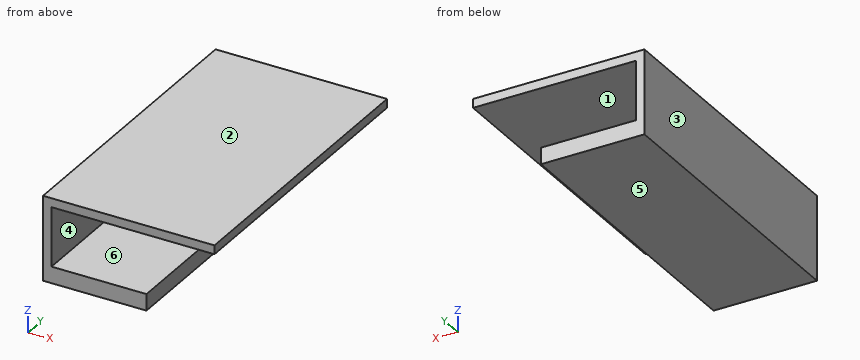
```python
from build123d import *

# Parameters (mm, degrees)
SKETCH2_W           = 106
SKETCH2_H           = 106
SKETCH2_R           = 4
SKETCH2_R_2         = 6
BOSS_EXTRUDE1_DEPTH = 25
SKETCH3_W           = 106
SKETCH3_H           = 106
SKETCH3_W_2         = 100
SKETCH3_H_2         = 100
BOSS_EXTRUDE2_DEPTH = 20
SKETCH5_W           = 3
SKETCH5_H           = 23
BOSS_EXTRUDE3_DEPTH = 20
SKETCH7_W           = 20
SKETCH7_H           = 3
BOSS_EXTRUDE4_DEPTH = 20
SKETCH9_R           = 9.905763918
CUT_EXTRUDE1_DEPTH  = 10
SKETCH10_W          = 10
SKETCH10_H          = 4
BOSS_EXTRUDE5_DEPTH = 10
SKETCH11_W          = 10
SKETCH11_H          = 4
BOSS_EXTRUDE6_DEPTH = 10
FILLET2_RADIUS      = 5
FILLET2_LENGTH      = 4
FILLET3_R           = 5
FILLET4_R           = 5
FILLET5_R           = 5
SKETCH13_R          = 1.6
CUT_EXTRUDE2_DEPTH  = 163.397660082
SKETCH14_W          = 35.96051594
SKETCH14_H          = 7.693498276
CUT_EXTRUDE3_DEPTH  = 30
BOSS_EXTRUDE7_DEPTH = 100
SKETCH21_W          = 151.44967638
SKETCH21_H          = 134.741704964
CUT_EXTRUDE6_DEPTH  = 187.257885739


with BuildPart() as part:
    # Sketch2 → Boss-Extrude1 (new body)
    with BuildSketch(Plane(origin=(0, 0, 0), x_dir=(1, 0, 0), z_dir=(0, 1, 0))):
        with Locations((53, 53)):
            Rectangle(SKETCH2_W, SKETCH2_H)
        with Locations(Location((18, 15, 0), (0, 0, 270))):
            Circle(SKETCH2_R, mode=Mode.SUBTRACT)
        with Locations(Location((92, 13.5, 0), (0, 0, 270))):
            Circle(SKETCH2_R_2, mode=Mode.SUBTRACT)
    extrude(amount=BOSS_EXTRUDE1_DEPTH)

    # Sketch3 → Boss-Extrude2 (add)
    with BuildSketch(Plane(origin=(0, 25, 0), x_dir=(1, 0, 0), z_dir=(0, 1, 0))):
        with Locations((53, 53)):
            Rectangle(SKETCH3_W, SKETCH3_H)
        with Locations((53, 53)):
            Rectangle(SKETCH3_W_2, SKETCH3_H_2, mode=Mode.SUBTRACT)
    extrude(amount=BOSS_EXTRUDE2_DEPTH)

    # Sketch5 → Boss-Extrude3 (add)
    with BuildSketch(Plane(origin=(0, 25, 0), x_dir=(1, 0, 0), z_dir=(0, 1, 0))):
        Polygon((3, 28), (3, 25), (32, 25), (32, 23), (35, 23), (35, 43), (32, 43), (32, 28), align=None)
        Polygon((83, 52.5), (83, 26.5), (76, 26.5), (76, 3), (73, 3), (73, 29.5), (80, 29.5), (80, 49.5), (73, 49.5), (73, 52.5), align=None)
        Polygon((3, 63), (3, 60), (25, 60), (25, 80), (22, 80), (22, 63), align=None)
        with Locations((59.5, 14.5)):
            Rectangle(SKETCH5_W, SKETCH5_H)
    extrude(amount=BOSS_EXTRUDE3_DEPTH)

    # Sketch7 → Boss-Extrude4 (add)
    with BuildSketch(Plane(origin=(0, 25, 0), x_dir=(1, 0, 0), z_dir=(0, 1, 0))):
        Polygon((50, 70.496538655), (53, 70.496538655), (53, 73.496538655), (53, 83.496538655), (50, 83.496538655), align=None)
        with Locations((63, 71.996538655)):
            Rectangle(SKETCH7_W, SKETCH7_H)
        Polygon((73, 70.496538655), (73, 52.5), (76, 52.5), (76, 82.5), (73, 82.5), (73, 73.496538655), align=None)
    extrude(amount=BOSS_EXTRUDE4_DEPTH)

    # Sketch9 → Cut-Extrude1 (cut)
    with BuildSketch(Plane(origin=(0, 25, 0), x_dir=(1, 0, 0), z_dir=(0, 1, 0))):
        with Locations(Location((92, 13.5, 0), (0, 0, 270))):
            Circle(SKETCH9_R)
    extrude(amount=-CUT_EXTRUDE1_DEPTH, mode=Mode.SUBTRACT)

    # Sketch10 → Boss-Extrude5 (add)
    with BuildSketch(Plane.XY):
        with Locations((53, 2)):
            Rectangle(SKETCH10_W, SKETCH10_H)
    extrude(amount=BOSS_EXTRUDE5_DEPTH)

    # Sketch11 → Boss-Extrude6 (add)
    with BuildSketch(Plane(origin=(0, 0, -106), x_dir=(-1, 0, 0), z_dir=(0, 0, -1))):
        with Locations((-53, 2)):
            Rectangle(SKETCH11_W, SKETCH11_H)
    extrude(amount=BOSS_EXTRUDE6_DEPTH)

    # Fillet2: full round fillet: the end face becomes a half cylinder, R = half its width
    fillet2_face = Plane((53, 2, -116), x_dir=(0, -1, 0), z_dir=(0, 0, -1))  # on the end face: x along it, z out of the body
    fillet2_slab = fillet2_face.offset(-FILLET2_RADIUS / 2) * Box(FILLET2_LENGTH, 2 * FILLET2_RADIUS, FILLET2_RADIUS, mode=Mode.PRIVATE)  # the body's end, R deep
    fillet2_round = Plane((53, 2, -111), x_dir=(0, 0, -1), z_dir=(0, -1, 0)) * Cylinder(FILLET2_RADIUS, FILLET2_LENGTH, mode=Mode.PRIVATE)  # its axis R under the face
    add(fillet2_slab - fillet2_round, mode=Mode.SUBTRACT)

    # Fillet3
    fillet3_edges = [part.edges().sort_by_distance(p)[0] for p in [
        (48, 2, -106),
        (58, 2, -106),
    ]]
    fillet(fillet3_edges, radius=FILLET3_R - 0.0001)  # a hair under: the kernel refuses the full size

    # Fillet4
    fillet4_edges = [part.edges().sort_by_distance(p)[0] for p in [
        (48, 2, 0),
        (58, 2, 0),
    ]]
    fillet(fillet4_edges, radius=FILLET4_R)

    # Fillet5
    fillet5_edges = [part.edges().sort_by_distance(p)[0] for p in [
        (48, 2, 10),
        (58, 2, 10),
    ]]
    fillet(fillet5_edges, radius=FILLET5_R - 0.0001)  # a hair under: the kernel refuses the full size

    # Sketch13 → Cut-Extrude2 (cut, through all)
    with BuildSketch(Plane(origin=(0, 4, 0), x_dir=(1, 0, 0), z_dir=(0, 1, 0))):
        with Locations(Location((53, -5, 0), (0, 0, 180))):
            Circle(SKETCH13_R)
        with Locations(Location((53, 111, 0), (0, 0, 180))):
            Circle(SKETCH13_R)
    extrude(amount=-CUT_EXTRUDE2_DEPTH, mode=Mode.SUBTRACT)

    # Sketch14 → Cut-Extrude3 (cut)
    with BuildSketch(Plane.XY):
        with Locations((88.01974203, 3.846749138)):
            Rectangle(SKETCH14_W, SKETCH14_H)
    extrude(amount=-CUT_EXTRUDE3_DEPTH, mode=Mode.SUBTRACT)

    # Sketch15 → Boss-Extrude7 (add)
    with BuildSketch(Plane(origin=(0, 45, 0), x_dir=(1, 0, 0), z_dir=(0, 1, 0))):
        Polygon((0, 28.5668375), (0, 0), (2.876085753, 0), (58, 0), (58, 3), (2.876085753, 3), (2.876085753, 23), (35, 23), (35, 28.5668375), align=None)
    extrude(amount=BOSS_EXTRUDE7_DEPTH)

    # Sketch21 → Cut-Extrude6 (cut, through all)
    with BuildSketch(Plane(origin=(0, 45, 0), x_dir=(1, 0, 0), z_dir=(0, 1, 0))):
        with Locations((51.832238557, 52.101721967)):
            Rectangle(SKETCH21_W, SKETCH21_H)
    extrude(amount=-CUT_EXTRUDE6_DEPTH, mode=Mode.SUBTRACT)


solid = part.part
```
Input: part model. Units: mm. Frame: model coordinates. Face numbers are marked on the shaded views. A direction names the side the tool comes from. Round coordinates to 2 decimals unless told otherwise and drop trailing zeros. Order: outer loops, then holes, each group sorted by start corner. A loop starts at its lowest first (then second) coordinate and runs counter-clockwise, first axis right, second up. Notation, with made-up numbers: (87.25, 0) - (95.25, 0) arc R10 ccw to (95.25, 15) - close; hole circle Ø9 at (16.5, 77). An arc over 180 degrees is marked (long way). Answer in a Markdown table with one row per item.
Item 1: Line query: line 1 (Z direction, x = 3.5, y = 77); line 2 (X direction, y = 60.5, z = -11.75); line 3 (Z direction, x = 52.5, y = 109.5). Output: solid intervals per line, ascending.
Model answer:
| item | result |
|---|---|
| line 1 | z = -28.57 to -23, -3 to 0 |
| line 2 | x = 0 to 2.88 |
| line 3 | z = -3 to 0 |
Item 2: Section query B-B (y = 90.5). Return the cut outline in (x, z), then the cut area to 3 significant figures.
Model answer:
| item | result |
|---|---|
| outline | (0, -28.57) - (35, -28.57) - (35, -23) - (2.88, -23) - (2.88, -3) - (58, -3) - (58, 0) - (0, 0) - close |
| area | 426 mm² |
Item 3: Mould query, pull axis Z, two halves, no side actions, for the marked faces 1, 2, 3 and 4. Classes: released by +Z, released by -Z, zero draft, split by the parting line, or undercut.
Model answer:
| item | result |
|---|---|
| face 1 | undercut |
| face 2 | released by +Z |
| face 3 | zero draft |
| face 4 | undercut |
Item 4: Reachability of the marked faces 5 and 6 from +Z, -Z, +X, -X, +Y, -Y: full face, straight path, thin tool, end or side. Return the list, or none.
Model answer:
| item | result |
|---|---|
| face 5 | -Z, +X, -X, +Y, -Y |
| face 6 | +X, +Y, -Y |
Item 5: Section query D-D (x = 41.5). Return the cut outline in (y, z).
Model answer:
| item | result |
|---|---|
| outline | (45, -3) - (145, -3) - (145, 0) - (45, 0) - close |
Item 6: Pin query (flat end, axial travel): pin 1 (3 mm diameter, centred on y = 109.5, z = -13, fed in from +X); pin 2 (6 mm diameter, centred on y = 87, z = -24.5, fed in from +X); pin 3 (1 mm diameter, centred on x = 49.5, y = 94, fed in from -Z); pin 4 (1.5 mm diameter, centred on x = 25.5, z = -5, fed in from +Y). Return the tip coordinate at first contact, or that it passes through.
Model answer:
| item | result |
|---|---|
| pin 1 | stops at x = 2.88 |
| pin 2 | stops at x = 35 |
| pin 3 | stops at z = -3 |
| pin 4 | passes through |
Item 7: Section query C-C (z = -11.5). Return the cut outline in (x, y), then the cut area to 3 significant figures.
Model answer:
| item | result |
|---|---|
| outline | (0, 45) - (2.88, 45) - (2.88, 145) - (0, 145) - close |
| area | 288 mm² |
Item 8: Section query A-A (x = 27). Return the cut outline in (y, z), then the cut area to 3 significant figures.
Model answer:
| item | result |
|---|---|
| outline | (45, -28.57) - (145, -28.57) - (145, -23) - (45, -23) - close; (45, -3) - (145, -3) - (145, 0) - (45, 0) - close |
| area | 857 mm² |
